from build123d import *

# Parameters (mm, degrees)
F0_W      = 100
F0_H      = 50
F1_DEPTH  = 5
F2_W      = 100
F2_H      = 50
F3_DEPTH  = 45
F4_W      = 12
F4_H      = 50
F5_DEPTH  = 3
F6_W      = 12
F6_H      = 50
F7_DEPTH  = 3
F8_D      = 3
F8_DEPTH  = 45
F8_TIP    = 0.9012909285
F11_D     = 2
F11_DEPTH = 20
F11_TIP   = 0.600860619


# Not quite as in the source:
# - a feature names something its author has since deleted; it is built from what else it names
# - the program builds the solid bodies; features that only make, move or delete a surface that nothing else refers to are left out


with BuildPart() as f1:
    # F0 (on Top) → F1 (new body)
    with BuildSketch(Plane.XY):
        with Locations((0.7340639085, 12.856667003)):
            Rectangle(F0_W, F0_H)
    extrude(amount=F1_DEPTH)

    # F2 (on face) → F3 (join)
    with BuildSketch(Plane.XY.offset(5)):
        with Locations((0.7340639085, 12.856667003)):
            Rectangle(F2_W, F2_H)
        with BuildLine():
            Line((-46.2659360915, -6.143332997), (-46.2659360915, 31.856667003))
            ThreePointArc((-46.2659360915, 31.856667003), (-44.144615748, 32.7353466595), (-43.2659360915, 34.856667003))
            Line((-43.2659360915, 34.856667003), (44.7340639085, 34.856667003))
            ThreePointArc((44.7340639085, 34.856667003), (45.6127435649, 32.7353466595), (47.7340639085, 31.856667003))
            Line((47.7340639085, 31.856667003), (47.7340639085, -6.143332997))
            ThreePointArc((47.7340639085, -6.143332997), (45.6127435649, -7.0220126534), (44.7340639085, -9.143332997))
            Line((44.7340639085, -9.143332997), (-43.2659360915, -9.143332997))
            ThreePointArc((-43.2659360915, -9.143332997), (-44.144615748, -7.0220126534), (-46.2659360915, -6.143332997))
        make_face(mode=Mode.SUBTRACT)
    extrude(amount=F3_DEPTH)

    # F4 (on face) → F5 (join)
    with BuildSketch(Plane.XZ.offset(12.143332997)):
        with Locations((-28.2659360915, 25)):
            Rectangle(F4_W, F4_H)
        with Locations((29.7340639085, 25)):
            Rectangle(F4_W, F4_H)
    extrude(amount=F5_DEPTH)

    # F6 (on face) → F7 (join)
    with BuildSketch(Plane(origin=(0, 37.856667003, 0), x_dir=(-1, 0, 0), z_dir=(0, 1, 0))):
        with Locations((-29.7340639085, 25)):
            Rectangle(F6_W, F6_H)
        with Locations((28.2659360915, 25)):
            Rectangle(F6_W, F6_H)
    extrude(amount=F7_DEPTH)

    # F8 (one way)
    with BuildSketch(Plane(origin=(0, 0, 5), x_dir=(1, 0, 0), z_dir=(0, 0, -1))):
        with Locations((-46.2659360915, -34.856667003), (-46.2659360915, 9.143332997), (47.7340639085, -34.856667003), (47.7340639085, 9.143332997)):
            Circle(F8_D / 2)
    extrude(amount=-F8_DEPTH, mode=Mode.SUBTRACT)
    with Locations(Plane(origin=(0, 0, 5), x_dir=(1, 0, 0), z_dir=(0, 0, -1))):
        with Locations((-46.2659360915, -34.856667003), (-46.2659360915, 9.143332997), (47.7340639085, -34.856667003), (47.7340639085, 9.143332997)):
            with Locations((0, 0, -(F8_DEPTH + F8_TIP / 2))):  # 118° drill point
                Cone(0, F8_D / 2, F8_TIP, mode=Mode.SUBTRACT)

    # F11
    with Locations(Plane(origin=(0, 0, 0), x_dir=(1, 0, 0), z_dir=(0, 0, -1))):
        with Locations((-42.2659360915, 5.143332997), (43.7340639085, 5.143332997), (43.7340639085, -30.856667003), (-42.2659360915, -30.856667003)):
            Hole(F11_D / 2, depth=F11_DEPTH)
            with Locations((0, 0, -(F11_DEPTH + F11_TIP / 2))):  # 118° drill point
                Cone(0, F11_D / 2, F11_TIP, mode=Mode.SUBTRACT)


solid = f1.part
Design review of the part built by this model. Coordinates are the model's own, in mm. A direction names the side the tool comes from. Coordinates: 2 decimals unless noted, no trailing zeros. Loops run counter-clockwise (first coordinate to the right, second up) from the corner with the lowest first, then second, coordinate; pieces in that order, holes last. Notation, with made-up numbers: (85, 20) - (144, 20) arc R19 ccw to (144, 26) - close; hole circle Ø9 at (11, 23). An arc over 180 degrees is marked (long way). Use CSV: the item, a comma, the result in double quotes. Start each with the question number.
1. Add section C-C on y = 21.5. Give the boundary of the cut face in (x, z), plus the area to 3 significant figures.
2. For faces 5 (the flat face through (-34.266, -14, 25)), 6 (the flat face through (-34.266, 39, 25)), 7 (the flat face through (35.734, 39, 25)), 8 (the cylindrical face through (-46.59, 36.32, 27.18)), list the 3-axis set-ups (+Z, -Z, +X, -X, +Y, -Y) from which the entire face can be reached by the end or side of a thin tool; tool diameter is ignored.
3. Add section B-B on x = -24.5. Give the boundary of the cut face in (y, z), plus the area to 3 significant figures.
4. To check wall thickness, follow probe 1 along X at (y, z) = (0, 30); probe 2 along Y at (x, z) = (5, 41); probe 3 along Y at (x, z) = (32.5, 6). State the ranges of each line that lie inside material, in increasing order.
5. Mouldability with a two-part tool opening along Y and no side actions: class faces 1 (the flat face through (-46, 35, 5)), 2 (the flat face through (30, 40.857, 25)), 3 (the flat face through (23.734, -14, 25)), 4 (the flat face through (-46, -9, 5)) as released by +Y, released by -Y, zero draft, split by the parting line, or undercut.
6. Clearance check with flat-ended pins moving along their axes: pin 1 (3 mm diameter, centred on x = 24, y = 0.5, fed in from +Z); pin 2 (2 mm diameter, centred on x = 1.5, y = 22.5, fed in from -Z); pin 3 (1.2 mm diameter, centred on x = 43.73, y = 30.86, fed in from -Z); pin 4 (1.5 mm diameter, centred on y = -14, z = 32, fed in from -X). State where each tip first meets the part, or that it passes through.
7. Add section A-A on z = 17. Count the separate pieces of the cut face and the enclosed holes in it, plus the area to 3 significant figures.
Resolved:
1,outline,"(-49.27, 0) - (50.73, 0) - (50.73, 50) - (47.73, 50) - (47.73, 5) - (-46.27, 5) - (-46.27, 50) - (-49.27, 50) - close"
1,area,"770 mm2"
2,face 5,"+Z, -Z, -X, -Y"
2,face 6,"+Z, -Z, -X, +Y"
2,face 7,"+Z, -Z, +X, +Y"
2,face 8,"+Z"
3,outline,"(-15.14, 0) - (40.86, 0) - (40.86, 50) - (34.86, 50) - (34.86, 5) - (-9.14, 5) - (-9.14, 50) - (-15.14, 50) - close"
3,area,"820 mm2"
4,probe 1,"-49.27 to -46.27, 47.73 to 50.73"
4,probe 2,"-12.14 to -9.14, 34.86 to 37.86"
4,probe 3,"-15.14 to -9.14, 34.86 to 40.86"
5,face 1,"undercut"
5,face 2,"released by +Y"
5,face 3,"zero draft"
5,face 4,"undercut"
6,pin 1,"z = 5"
6,pin 2,"z = 0"
6,pin 3,"through"
6,pin 4,"x = -34.27"
7,separate pieces,"1"
7,enclosed holes,"5"
7,area,"1,010 mm2"
